from build123d import *

# Parameters (mm, degrees)
SKETCH_W        = 80
SKETCH_H        = 20
SKETCH_R        = 3.2
PAD_DEPTH       = 22
SKETCH001_R     = 11.1
POCKET_DEPTH    = 8
SKETCH002_R     = 6
SKETCH002_R_2   = 8
POCKET001_DEPTH = 20


with BuildPart() as part:
    # Sketch → Pad (new body)
    with BuildSketch(Plane.XY):
        with Locations((40, 10)):
            Rectangle(SKETCH_W, SKETCH_H)
        with Locations((20, 15)):
            Circle(SKETCH_R, mode=Mode.SUBTRACT)
        with Locations((20, 5)):
            Circle(SKETCH_R, mode=Mode.SUBTRACT)
        with Locations((60, 15)):
            Circle(SKETCH_R, mode=Mode.SUBTRACT)
        with Locations((60, 5)):
            Circle(SKETCH_R, mode=Mode.SUBTRACT)
    extrude(amount=PAD_DEPTH)

    # Sketch001 (on Face3 of Pad) → Pocket (cut)
    with BuildSketch(Plane.XZ):
        with Locations((40, 11)):
            Circle(SKETCH001_R)
    extrude(amount=-POCKET_DEPTH, mode=Mode.SUBTRACT)

    # Sketch002 (on Face1 of Pocket) → Pocket001 (cut)
    with BuildSketch(Plane(origin=(0, 20, 0), x_dir=(-1, 0, 0), z_dir=(0, 1, 0))):
        with Locations((-72, 11)):
            Circle(SKETCH002_R)
        with Locations((-8, 11)):
            Circle(SKETCH002_R)
        with Locations((-40, 11)):
            Circle(SKETCH002_R_2)
    extrude(amount=-POCKET001_DEPTH, mode=Mode.SUBTRACT)


solid = part.part
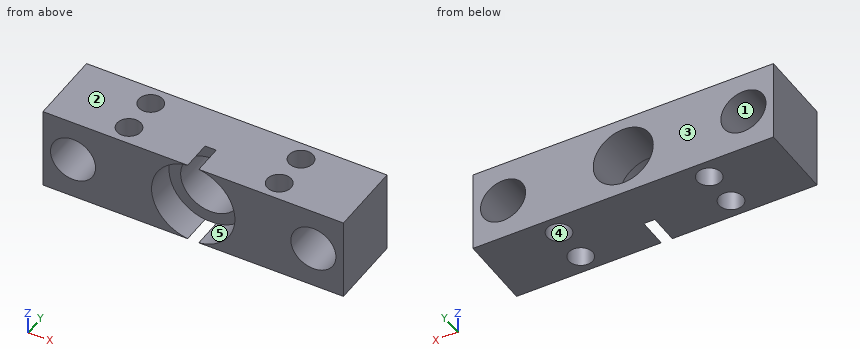
Geometry: final body of the model. Coordinates: model frame, mm. Face numbers are marked on the shaded views. A direction names the side the tool comes from. Give positions to 0.01 mm unless a question says otherwise; leave off trailing zeros. Order: outer loops, then holes, each group sorted by start corner. A loop starts at its lowest first (then second) coordinate and runs counter-clockwise, first axis right, second up. Notation, with made-up numbers: (53, 66.5) -> (97, 66.5) arc R20 cw to (97, 77.5) -> close; hole circle Ø3 at (59.25, 83.25). An arc over 180 degrees is marked (long way). Put each result on its own line as item: value.
Q1. Section D-D, the plane x = 11. Return loops of the section in (y, z), then the cut area to 3 significant figures.
Here are the results:
outline: (0, 0) -> (20, 0) -> (20, 5.8) -> (0, 5.8) -> close; (0, 16.2) -> (20, 16.2) -> (20, 22) -> (0, 22) -> close
area: 232 mm^2
Q2. Material intervals for L1, parallel to Y at x = 20, z = 8; L2, parallel to Z at x = 72, y = 15.75; L3, parallel to X at y = 6, z = 13, sorted ascending.
Here are the results:
L1: y = 0 to 1.8, 8.2 to 11.8, 18.2 to 20
L2: z = 0 to 5, 17 to 22
L3: x = 0 to 2.34, 13.66 to 16.96, 23.04 to 29.08, 50.92 to 56.96, 63.04 to 66.34, 77.66 to 80
Q3. Reachability of the marked faces 4 and 5 from +Z, -Z, +X, -X, +Y, -Y: full face, straight path, thin tool, end or side. Return the list, or none.
Here are the results:
face 4: +Z, -Z
face 5: -Y
Q4. Section A-A, the plane z = 11. Return loops of the section in (x, y), then the cut area to 3 significant figures.
Here are the results:
outline: (0, 0) -> (2, 0) -> (2, 20) -> (0, 20) -> close; (14, 0) -> (28.9, 0) -> (28.9, 8) -> (32, 8) -> (32, 20) -> (14, 20) -> close; (48, 8) -> (51.1, 8) -> (51.1, 0) -> (66, 0) -> (66, 20) -> (48, 20) -> close; (78, 0) -> (80, 0) -> (80, 20) -> (78, 20) -> close; hole circle Ø6.4 at (20, 5); hole circle Ø6.4 at (20, 15); hole circle Ø6.4 at (60, 5); hole circle Ø6.4 at (60, 15)
area: 622 mm^2
Q5. Section B-B, the plane x = 20. Return loops of the section in (y, z), then the cut area to 3 significant figures.
Here are the results:
outline: (0, 0) -> (1.8, 0) -> (1.8, 22) -> (0, 22) -> close; (8.2, 0) -> (11.8, 0) -> (11.8, 22) -> (8.2, 22) -> close; (18.2, 0) -> (20, 0) -> (20, 22) -> (18.2, 22) -> close
area: 158 mm^2
Q6. Section C-C, the plane y = 5. Return loops of the section in (x, z).
Here are the results:
outline: (0, 0) -> (16.8, 0) -> (16.8, 22) -> (0, 22) -> close; (23.2, 0) -> (38.51, 0) arc R11.1 cw to (38.51, 22) -> (23.2, 22) -> close; (41.49, 0) -> (56.8, 0) -> (56.8, 22) -> (41.49, 22) arc R11.1 cw to start; (63.2, 0) -> (80, 0) -> (80, 22) -> (63.2, 22) -> close; hole circle Ø12 at (8, 11); hole circle Ø12 at (72, 11)
Q7. Draft query along Z for the marked faces 1, 2 and 3. Return one class per face: released by +Z, released by -Z, zero draft, split by the parting line, or undercut.
Here are the results:
face 1: undercut
face 2: released by +Z
face 3: zero draft
